from build123d import *

# Parameters (mm, degrees)
F1_DEPTH = 3
F3_DEPTH = 1143.9908999712


# Not quite as in the source:
# - ends of sketch curves that miss each other by under 0.0002 mm in the source are joined
# - a feature names something its author has since deleted; it is built from what else it names


with BuildPart() as f1:
    # F0 (on Right) → F1 (new body)
    with BuildSketch(Plane.YZ):
        Polygon((-1080.583592135, 376.3379858925), (7.416407865, 22.8253563911), (13.9057647469, 42.7975432333), (-1074.0942352531, 396.3101727347), align=None)
        Polygon((-1088, 353.5126295014), (0, 0), (6.4893568819, 19.9721868422), (-1081.5106431181, 373.4848163436), align=None)
        Polygon((-1081.5106431181, 373.4848163436), (6.4893568819, 19.9721868422), (6.9528823734, 21.3987716166), (-1081.0471176266, 374.911401118), align=None)
        Polygon((-1081.0471176266, 374.911401118), (6.9528823734, 21.3987716166), (7.416407865, 22.8253563911), (-1080.583592135, 376.3379858925), align=None)
    extrude(amount=-F1_DEPTH)

    # F2 (on face) → F3 (join, through all)
    with BuildSketch(Plane(origin=(0, -1088, 353.5126295014), x_dir=(1, 0, 0), z_dir=(0, -0.9510565163, 0.3090169944))):
        Polygon((-60.7660203681, 22.5), (-57.3180156743, 22.5), (-3, 22.5), (-3, 24), (-60.7660203681, 24), align=None)
        Polygon((-3, 21), (-3, 22.5), (-3.1967548982, 21), align=None)
        Polygon((-3.1967548982, 21), (-3, 22.5), (-6.2963244545, 21), align=None)
        Polygon((-3, 22.5), (-57.3180188703, 22.5), (-57.5147689745, 21), (-6.2963244545, 21), align=None)
        Polygon((-57.5147689745, 21), (-57.3180140763, 22.5), (-60.7660203681, 22.5), (-60.7660203681, 21), align=None)
    extrude(amount=-F3_DEPTH)


solid = f1.part
Geometry: final body of the model. Coordinates: model frame, mm. A direction names the side the tool comes from. Give positions to 0.01 mm unless a question says otherwise; leave off trailing zeros. Loops run counter-clockwise (first coordinate to the right, second up) from the corner with the lowest first, then second, coordinate; pieces in that order, holes last. Notation, with made-up numbers: M -39.75,-24 L -11.75,-24 A30 cw -11.75,12 Z; hole C 0.25,-1 d10. An arc over 180 degrees is marked long. Put each result on its own line as item: value. Start each with the question number.
1) Ray query, line 1 along Z through (x, y) = (-56, -83); line 2 along X through (y, z) = (-368, 145.5); line 3 along Z through (x, y) = (-51.5, -804.5). Return the intervals inside material, ascending.
2) Access query for faces 1 (the flat face through (-32.287, -545.127, 199.203)), 2 (the flat face through (0, -540, 199)), 3 (the flat face through (-3, -536, 210)). Directions: +Z, -Z, +X, -X, +Y, -Y. A direction counts if a zero-diameter tool reaches every point of the face in a straight line with its end or side. Return the directions, or none.
3) Cut plane C-C (x = -38). Output: boundary loops of the cut face in (y, z), then the cut area to 3 significant figures.
4) Cut plane A-A (z = 123). Output: boundary loops of the cut face in (x, y), then the cut area to 3 significant figures.
5) Contact query for flat-ended pins moving along their axis: pin 1 (6 mm diameter, centred on x = -29, y = -958, fed in from +Z); pin 2 (10 mm diameter, centred on x = -53, y = -749, fed in from +Z); pin 3 (8 mm diameter, centred on x = -40.5, y = -480.5, fed in from -Z). Output: stop coordinate, or through.
6) Cut plane B-B (y = -286.5). Output: boundary loops of the cut face in (x, z), then the cut area to 3 significant figures.
Verdict:
1. line 1: 49.05 to 52.2
1. line 2: -3 to 0
1. line 3: 283.48 to 286.63
2. face 1: -Z, -X, -Y
2. face 2: +Z, -Z, +X, +Y, -Y
2. face 3: +Z, -X, +Y
3. outline: M -1081.51,373.48 L 6.49,19.97 L 7.42,22.83 L -1080.58,376.34 Z
3. area: 3,430 mm2
4. outline: M -60.77,-310.6 L -3,-310.6 L -3,-378.56 L 0,-378.56 L 0,-232.93 L -3,-232.93 L -3,-300.89 L -60.77,-300.89 Z
4. area: 998 mm2
5. pin 1: z = 337.48
5. pin 2: z = 270.22
5. pin 3: z = 176.9
6. outline: M -60.77,115.17 L -3,115.17 L -3,93.09 L 0,93.09 L 0,140.41 L -3,140.41 L -3,118.32 L -60.77,118.32 Z
6. area: 324 mm2
